Could you check a few things on this model? Use its own coordinates, in mm. A direction names the side the tool comes from. Give positions to 0.01 mm unless a question says otherwise; leave off trailing zeros. Loops run counter-clockwise (first coordinate to the right, second up) from the corner with the lowest first, then second, coordinate; pieces in that order, holes last. Notation, with made-up numbers: (47, -2.5) -> (51, -2.5) arc R16 ccw to (51, 5.5) -> close; hole circle Ø4 at (-33, 27.5). An arc over 180 degrees is marked (long way). Put each result on its own line as item: value.
Autodesk Inventor part; units mm, degrees
ref_plane "YZ Plane" through (0, 0, 0) normal (1, 0, 0) x (0, 1, 0)
ref_plane "XZ Plane" through (0, 0, 0) normal (0, 1, 0) x (-1, 0, 0)
ref_plane "XY Plane" through (0, 0, 0) normal (0, 0, 1) x (1, 0, 0)
sketch "Sketch1" plane through (0, 0, 0) normal (0, 0, 1) x (1, 0, 0)
  line L0 (0, -7.3524) -> (0, 22.6476) construction
  line L1 (1.5, -7.3524) -> (1.5, 22.6476)
  line L2 (-1.5, 22.6476) -> (-1.5, -7.3524)
  arc A0 (-1.5, -7.3524) -> (1.5, -7.3524) centre (0, -7.3524) ccw
  arc A1 (1.5, 22.6476) -> (-1.5, 22.6476) centre (0, 22.6476) ccw
  line L3 (-2.5, -7.3524) -> (-2.5, 22.6476)
  arc A2 (2.5, 22.6476) -> (-2.5, 22.6476) centre (0, 22.6476) ccw
  line L4 (2.5, 22.6476) -> (2.5, -7.3524)
  arc A3 (-2.5, -7.3524) -> (2.5, -7.3524) centre (0, -7.3524) ccw
  line L5 (-5.6, 22.6476) -> (-5.6, -7.3524)
  arc A4 (-5.6, -7.3524) -> (5.6, -7.3524) centre (0, -7.3524) ccw
  line L6 (5.6, -7.3524) -> (5.6, 22.6476)
  arc A5 (5.6, 22.6476) -> (-5.6, 22.6476) centre (0, 22.6476) ccw
  line L7 (-4.1, 22.6476) -> (-4.1, -7.3524)
  arc A6 (-4.1, -7.3524) -> (4.1, -7.3524) centre (0, -7.3524) ccw
  line L8 (4.1, -7.3524) -> (4.1, 22.6476)
  arc A7 (4.1, 22.6476) -> (-4.1, 22.6476) centre (0, 22.6476) ccw
  point P0 (0, 0)
  point P1 (0, 7.6476)
  point P2 (0, 26.7476)
  point P3 (0, -11.4524)
  point P4 (-4.1, 7.6476)
  point P5 (-4.1, 22.6476)
  point P6 (4.1, 7.6476)
  point P7 (-4.1, 7.6476)
  dimension "d0" = 30
  dimension "d1" = 3
  dimension "d2" = 1
  dimension "d3" = 3.1
  dimension "d10" = 1.6
  dimension "d16" = 15
extrude "Extrusion1" add sketch "Sketch1" along normal blind 2.5 contours A0 L2 A1 L1
extrude "Extrusion2" add sketch "Sketch1" against normal blind 0.6 contours A5 L6 A4 L5 | A7 L8 A6 L7
extrude "Extrusion3" add sketch "Sketch1" against normal blind 4 contours A0 L2 A1 L1 | L3 A2 L4 A3
hole "Hole1" at (0, 26.7476, 0) at (0, -11.4524, 0) at (-4.1, -7.3524, 0) at (-4.1, 7.6476, 0) at (-4.1, 22.6476, 0) at (4.1, -7.3524, 0) at (4.1, 7.6476, 0) at (4.1, 22.6476, 0) direction (0, 0, -1) diameter 1.6 end through all both
chamfer "Chamfer1" distance 1 angle 45 4 edges at (0, -9.8524, -4) (-2.5, 7.6476, -4) (0, 25.1476, -4) (2.5, 7.6476, -4)
sketch "Sketch2" plane through (-2.5, -7.3524, -0.6) normal (-1, 0, 0) x (0, 0, 1)
  line L0 (-2.4, 0) -> (-2.4, 30)
  line L1 (0, 0) -> (-2.4, 0)
  line L2 (0, 30) -> (0, 0)
  line L3 (0, 30) -> (-2.4, 30)
  line L4 (-2.4, 30) -> (-2.4, 0)
  line L5 (-2.4, 1.2) -> (-2.4, 3.2) construction
  line L6 (-1.9, 1.2) -> (-1.9, 3.2)
  line L7 (-2.9, 3.2) -> (-2.9, 1.2)
  arc A0 (-2.9, 1.2) -> (-1.9, 1.2) centre (-2.4, 1.2) ccw
  arc A1 (-1.9, 3.2) -> (-2.9, 3.2) centre (-2.4, 3.2) ccw
  line L8 (-1.4, 1.2) -> (-1.4, 3.2)
  arc A2 (-1.4, 3.2) -> (-3.4, 3.2) centre (-2.4, 3.2) ccw
  line L9 (-3.4, 3.2) -> (-3.4, 1.2)
  arc A3 (-3.4, 1.2) -> (-1.4, 1.2) centre (-2.4, 1.2) ccw
  circle A4 centre (-2.4, 1.2) radius 0.5
  circle A5 centre (-2.4, 3.2) radius 0.5
  circle A6 centre (-2.4, 2.2) radius 0.5
  point P0 (0.6, 7.3524)
  dimension "d31" = 2
  dimension "d32" = 1
  dimension "d33" = 1.2
  dimension "d34" = 0.5
extrude "Extrusion5" add sketch "Sketch2" against normal blind 1 contours A3 L9 A2 L0 A1 L7 A0 | L0 A0 L6 A1 A2 L8 A3
extrude "Extrusion6" add sketch "Sketch2" along normal mid plane 8 contours A0 A4 L0 | L0 A4 A0 | A6 L0 | L0 A6 | A5 A1 L0 | L0 A1 A5
properties part number "ASSEMBLY_Regolith_level_sensor" material "Aluminum 6061"
1. If we section it at C-C (x = 3.75): List the corners of the cut face in (y, z) for me.
Recorded:
outline: (-11.51, -0.6) -> (-8.07, -0.6) -> (-8.07, 0) -> (-11.51, 0) -> close; (-6.63, -0.6) -> (6.93, -0.6) -> (6.93, 0) -> (-6.63, 0) -> close; (8.37, -0.6) -> (21.93, -0.6) -> (21.93, 0) -> (8.37, 0) -> close; (23.37, -0.6) -> (26.81, -0.6) -> (26.81, 0) -> (23.37, 0) -> close
2. I'm going to push flat-ended pins straight in: pin 1 (0.6 mm diameter, centred on x = -2.5, y = -4.5, fed in from +Z); pin 2 (2.5 mm diameter, centred on y = 9, z = -2, fed in from +X); pin 3 (1.4 mm diameter, centred on x = 4.1, y = -7.35, fed in from +Z); pin 4 (1.5 mm diameter, centred on y = 13, z = -1, fed in from -X). Where does each tip first touch, or does it pass through?
Recorded:
pin 1: stops at z = 0
pin 2: stops at x = 2.5
pin 3: passes through
pin 4: stops at x = -5.6
3. For faces 4 (the face through (-1.5, 8, 1)), 5 (the face through (-0.05, -9.85, -1.78)), 6 (the face through (4.065, 8.447, -0.304)), 7 (the face through (-1.9, -7.2, -3.6)), 8 (the face through (0, 8, -4)), which set-ups out of +Z, -Z, +X, -X, +Y, -Y let a thin tool reach every point of the face, with its end or its side?
Recorded:
face 4: +Z, -X, +Y, -Y
face 5: -Z, -Y
face 6: +Z, -Z
face 7: -Z, -X, -Y
face 8: -Z, +X, -X, +Y, -Y
4. I need wall thicknesses on line 1 (Y direction, x = 0, z = -0.35); line 2 (Y direction, x = -4.1, z = -0.4); line 3 (Z direction, x = -4, y = 25). Which ranges of each line are inside material? Lowest first, please.
Recorded:
line 1: y = -12.95 to -12.25, -10.65 to 25.95, 27.55 to 28.25
line 2: y = -11.17 to -8.15, -6.55 to 6.85, 8.45 to 21.85, 23.45 to 26.46
line 3: z = -0.6 to 0
5. Thinking about a two-plate mould opening in Y: for faces 1 (the face through (-2.118, -6.717, -3.825)), 2 (the face through (1.5, 7, 1)), 3 (the face through (-3.61, 8.28, -0.3)), which applies, pulls with the +Y half, pulls with the -Y half, needs draft (parallel to the pull), parting line crosses it, or undercut?
Recorded:
face 1: pulls with the -Y half
face 2: needs draft
face 3: undercut
6. If we section it at B-B (y = -0.5): List the corners of the cut face in (x, z) for me.
Recorded:
outline: (-5.6, -0.6) -> (-2.5, -0.6) -> (-2.5, -3) -> (-1.5, -4) -> (1.5, -4) -> (2.5, -3) -> (2.5, -0.6) -> (5.6, -0.6) -> (5.6, 0) -> (1.5, 0) -> (1.5, 2.5) -> (-1.5, 2.5) -> (-1.5, 0) -> (-5.6, 0) -> close
